Verification items for the finished model (mm, model axes). A direction names the side the tool comes from. Give positions to 0.01 mm unless a question says otherwise; leave off trailing zeros. Answer as a JSON object with one key per item and string values.
```python
from build123d import *

# Parameters (mm, degrees)
F0_R     = 3.175
F1_DEPTH = 0.254
F2_DEPTH = 21.59
F2_TAPER = 5


# Not quite as in the source:
# - a feature names something its author has since deleted; it is built from what else it names


with BuildPart() as f1:
    # F0 (on Front) → F1 (new body)
    with BuildSketch(Plane.XZ):
        with BuildLine():
            Line((-128.27, -165.1), (128.27, -165.1))
            ThreePointArc((128.27, -165.1), (132.7601280605, -163.2401280605), (134.62, -158.75))
            Line((134.62, -158.75), (134.62, 158.75))
            ThreePointArc((134.62, 158.75), (132.7601280605, 163.2401280605), (128.27, 165.1))
            Line((128.27, 165.1), (-128.27, 165.1))
            ThreePointArc((-128.27, 165.1), (-132.7601280605, 163.2401280605), (-134.62, 158.75))
            Line((-134.62, 158.75), (-134.62, -158.75))
            ThreePointArc((-134.62, -158.75), (-132.7601280605, -163.2401280605), (-128.27, -165.1))
        make_face()
        with Locations((-76.2, -160.02)):
            Circle(F0_R, mode=Mode.SUBTRACT)
        with Locations((0, -160.02)):
            Circle(F0_R, mode=Mode.SUBTRACT)
        with Locations((78.74, -160.02)):
            Circle(F0_R, mode=Mode.SUBTRACT)
        with Locations((-76.2, 158.75)):
            Circle(F0_R, mode=Mode.SUBTRACT)
        with Locations((-8.5018249229, 158.75)):
            Circle(F0_R, mode=Mode.SUBTRACT)
        with BuildLine():
            ThreePointArc((119.38, -144.78), (117.5201280605, -149.2701280605), (113.03, -151.13))
            Line((113.03, -151.13), (76.2, -151.13))
            Line((76.2, -151.13), (-76.2, -151.13))
            Line((-76.2, -151.13), (-113.03, -151.13))
            ThreePointArc((-113.03, -151.13), (-117.5201280605, -149.2701280605), (-119.38, -144.78))
            Line((-119.38, -144.78), (-119.38, 144.78))
            ThreePointArc((-119.38, 144.78), (-117.5201280605, 149.2701280605), (-113.03, 151.13))
            Line((-113.03, 151.13), (-76.2, 151.13))
            Line((-76.2, 151.13), (76.2, 151.13))
            Line((76.2, 151.13), (113.03, 151.13))
            ThreePointArc((113.03, 151.13), (117.5201280605, 149.2701280605), (119.38, 144.78))
            Line((119.38, 144.78), (119.38, -144.78))
        make_face(mode=Mode.SUBTRACT)
        with Locations((67.6981750771, 158.75)):
            Circle(F0_R, mode=Mode.SUBTRACT)
        with BuildLine():
            Line((76.2, -151.13), (113.03, -151.13))
            ThreePointArc((113.03, -151.13), (117.5201280605, -149.2701280605), (119.38, -144.78))
            Line((119.38, -144.78), (119.38, 144.78))
            ThreePointArc((119.38, 144.78), (117.5201280605, 149.2701280605), (113.03, 151.13))
            Line((113.03, 151.13), (76.2, 151.13))
            Line((76.2, 151.13), (-76.2, 151.13))
            Line((-76.2, 151.13), (-113.03, 151.13))
            ThreePointArc((-113.03, 151.13), (-117.5201280605, 149.2701280605), (-119.38, 144.78))
            Line((-119.38, 144.78), (-119.38, -144.78))
            ThreePointArc((-119.38, -144.78), (-117.5201280605, -149.2701280605), (-113.03, -151.13))
            Line((-113.03, -151.13), (-76.2, -151.13))
            Line((-76.2, -151.13), (76.2, -151.13))
        make_face()
    extrude(amount=F1_DEPTH)

    # F0 (on Front) → F2 (join)
    with BuildSketch(Plane.XZ):
        with BuildLine():
            Line((76.2, -151.13), (113.03, -151.13))
            ThreePointArc((113.03, -151.13), (117.5201280605, -149.2701280605), (119.38, -144.78))
            Line((119.38, -144.78), (119.38, 144.78))
            ThreePointArc((119.38, 144.78), (117.5201280605, 149.2701280605), (113.03, 151.13))
            Line((113.03, 151.13), (76.2, 151.13))
            Line((76.2, 151.13), (-76.2, 151.13))
            Line((-76.2, 151.13), (-113.03, 151.13))
            ThreePointArc((-113.03, 151.13), (-117.5201280605, 149.2701280605), (-119.38, 144.78))
            Line((-119.38, 144.78), (-119.38, -144.78))
            ThreePointArc((-119.38, -144.78), (-117.5201280605, -149.2701280605), (-113.03, -151.13))
            Line((-113.03, -151.13), (-76.2, -151.13))
            Line((-76.2, -151.13), (76.2, -151.13))
        make_face()
    extrude(amount=F2_DEPTH, taper=F2_TAPER)


solid = f1.part
```
Q1. Gauge pin test, flat ends, axial feed: pin 1 Ø10 at (x, z) = (-76.2, -160.02) entering from -Y; pin 2 Ø10 at (x, y) = (46.5, -10.5) entering from -Z; pin 3 Ø2 at (x, y) = (-35.5, -16) entering from +Z. Record the tip position at first contact, or that the pin passes through.
Resolved:
{"pin 1": "stops at y = -0.25", "pin 2": "stops at z = -150.65", "pin 3": "stops at z = 149.82"}
Q2. Material ranges on L1, parallel to X at y = -0.2, z = 158.75 (3 decimals); L2, parallel to Z at x = -76.2, y = -0.2 (3 decimals); L3, parallel to Y at x = -121.5, z = 121, recorded low to high.
Resolved:
{"L1": "x = -134.62 to -79.375, -73.025 to -11.677, -5.327 to 64.523, 70.873 to 134.62", "L2": "z = -165.1 to -163.195, -156.845 to 155.575, 161.925 to 165.1", "L3": "y = -0.25 to 0"}
Q3. Tool access check on faces 1 (the face through (2, -21.59, 2)), 2 (the face through (-120, -0.254, 1)). Record the directions out of +Z, -Z, +X, -X, +Y, -Y that give a thin tool (end or side, any length) a straight path to the whole face; none if there is none.
Resolved:
{"face 1": "+Z, -Z, +X, -X, -Y", "face 2": "-Y"}
